Here's how the part is built. I have some questions about the finished solid (model axes, mm). Round coordinates to 2 decimals unless told otherwise and drop trailing zeros. Write each loop counter-clockwise with the first axis right and the second up, starting at its lowest first coordinate (ties: lowest second). Pieces come first, ordered by that corner, then holes. Notation, with made-up numbers: M -10.5,-4.5 L 48.5,-4.5 A3 ccw 48.5,0.5 Z; hole C 56.25,32 d1. An arc over 180 degrees is marked long. Use a Markdown table: item, result. Add a question column.
```python
from build123d import *

# Parameters (mm, degrees)
SKETCH1_W           = 90
SKETCH1_H           = 8.5
SKETCH1_R           = 1.47
BOSS_EXTRUDE1_DEPTH = 3.18
SKETCH2_R           = 1.47
CUT_EXTRUDE1_DEPTH  = 91.456411602
FILLET1_R           = 2


with BuildPart() as part:
    # Sketch1 → Boss-Extrude1 (new body)
    with BuildSketch(Plane.XY):
        with Locations((45, 4.25)):
            Rectangle(SKETCH1_W, SKETCH1_H)
        with Locations(Location((87.5, 4.25, 0), (0, 0, 180))):
            Circle(SKETCH1_R, mode=Mode.SUBTRACT)
    extrude(amount=BOSS_EXTRUDE1_DEPTH)

    # Sketch2 → Cut-Extrude1 (cut, through all)
    with BuildSketch(Plane.XY.offset(3.18)):
        with Locations((45, 4.25)):
            Circle(SKETCH2_R)
    extrude(amount=-CUT_EXTRUDE1_DEPTH, mode=Mode.SUBTRACT)

    # Fillet1
    fillet1_edges = [part.edges().sort_by_distance(p)[0] for p in [
        (90, 8.5, 1.59),
        (90, 0, 1.59),
    ]]
    fillet(fillet1_edges, radius=FILLET1_R)


solid = part.part
```
Item 1: I need wall thicknesses on probe 1 along Y at (x, z) = (87.5, 1); probe 2 along X at (y, z) = (5, 0.3); probe 3 along X at (y, z) = (3, 1.7). Which ranges of each line are inside material? Lowest first, please. Write a range as from..to.
Item 2: If we mould it in two halves opening along X, with no side actions, what happens to faces 1 (the face through (90, 4, 2)), 2 (the face through (0, 4, 2)), 3 (the face through (86.14, 4.81, 1.57)), 4 (the face through (44, 6, 0))? For each: +X half, -X half, draft (parallel to the pull), parting line (faces both ways), or undercut.
Item 3: Imagine slicing it at C-C on y = 4.25. List the corners of the cut face in (x, z) for me.
Item 4: Imagine slicing it at B-B on x = 45. List the corners of the cut face in (y, z) for me, plus the area to 3 significant figures.
Item 5: Imagine slicing it at A-A on z = 1.55. List the corners of the cut face in (x, y) for me, plus the area to 3 significant figures.
The answers:
| question | item | result |
|---|---|---|
| 1 | probe 1 | 0..2.78, 5.72..8.5 |
| 1 | probe 2 | 0..43.74, 46.26..86.24, 88.76..90 |
| 1 | probe 3 | 0..44.23, 45.77..86.73, 88.27..90 |
| 2 | face 1 | +X half |
| 2 | face 2 | -X half |
| 2 | face 3 | undercut |
| 2 | face 4 | draft |
| 3 | outline | M 0,0 L 43.53,0 L 43.53,3.18 L 0,3.18 Z; M 46.47,0 L 86.03,0 L 86.03,3.18 L 46.47,3.18 Z; M 88.97,0 L 90,0 L 90,3.18 L 88.97,3.18 Z |
| 4 | outline | M 0,0 L 2.78,0 L 2.78,3.18 L 0,3.18 Z; M 5.72,0 L 8.5,0 L 8.5,3.18 L 5.72,3.18 Z |
| 4 | area | 17.7 mm² |
| 5 | outline | M 0,0 L 88,0 A2 ccw 90,2 L 90,6.5 A2 ccw 88,8.5 L 0,8.5 Z; hole C 45,4.25 d2.94; hole C 87.5,4.25 d2.94 |
| 5 | area | 750 mm² |
